Geometry check sheet. Reference: drawing and pictorial views, mm from the part's lowest x, y, z. Round coordinates to 2 decimals unless told otherwise and drop trailing zeros. Order: outer loops, then holes, each group sorted by start corner. A loop starts at its lowest first (then second) coordinate and runs counter-clockwise, first axis right, second up. Notation, with made-up numbers: (47, 43.5) -> (74, 43.5) arc R23 cw to (74, 58.5) -> close; hole circle Ø6 at (61.5, 40.5). An arc over 180 degrees is marked (long way). Put each result on its own line as item: value.
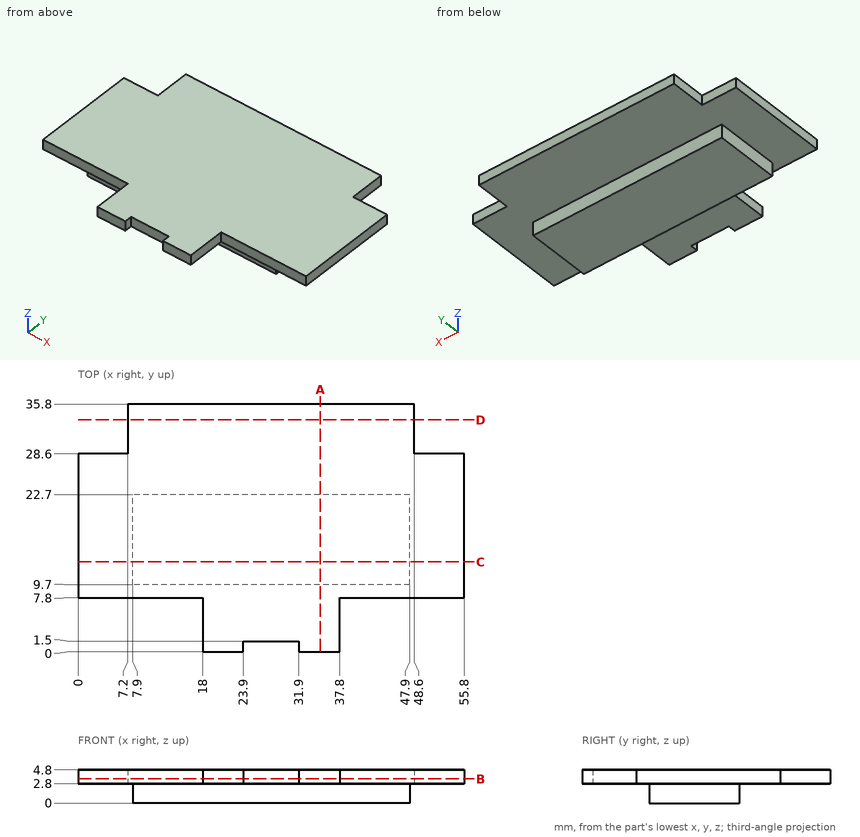
Item 1: Depth check by flat-ended pin: pin 1 Ø6 at (x, y) = (42, 15) entering from -Z; pin 2 Ø2 at (y, z) = (5.5, 3.5) entering from -X; pin 3 Ø1.6 at (y, z) = (3, 3.5) entering from +X; pin 4 Ø0.6 at (x, z) = (2, 4) entering from +Y. Enter the tip coordinate at first touch or a pass-through.
Geometry check:
pin 1: z = 0
pin 2: x = 18
pin 3: x = 37.8
pin 4: y = 28.6
Item 2: Sectioned sample at D-D, the plane y = 33.5. Record the boundary of the cut face in (x, z), then the cut area to 3 significant figures.
Geometry check:
outline: (7.2, 2.8) -> (48.6, 2.8) -> (48.6, 4.8) -> (7.2, 4.8) -> close
area: 82.8 mm2
Item 3: Material ranges on line 1 along Z through (x, y) = (29, 7); line 2 along Y through (x, z) = (38.5, 3.4); line 3 along X through (y, z) = (17.5, 1), recorded low to high.
Geometry check:
line 1: 2.8 to 4.8
line 2: 7.8 to 35.8
line 3: 7.9 to 47.9
Item 4: Sectioned sample at B-B, the plane z = 3.5. Record the boundary of the cut face in (x, y), then the cut area to 3 significant figures.
Geometry check:
outline: (0, 7.8) -> (18, 7.8) -> (18, 0) -> (23.9, 0) -> (23.9, 1.5) -> (31.9, 1.5) -> (31.9, 0) -> (37.8, 0) -> (37.8, 7.8) -> (55.8, 7.8) -> (55.8, 28.6) -> (48.6, 28.6) -> (48.6, 35.8) -> (7.2, 35.8) -> (7.2, 28.6) -> (0, 28.6) -> close
area: 1,600 mm2
Item 5: Sectioned sample at C-C, the plane y = 13. Record the boundary of the cut face in (x, z).
Geometry check:
outline: (0, 2.8) -> (7.9, 2.8) -> (7.9, 0) -> (47.9, 0) -> (47.9, 2.8) -> (55.8, 2.8) -> (55.8, 4.8) -> (0, 4.8) -> close
Item 6: Sectioned sample at A-A, the plane x = 35. Record the boundary of the cut face in (y, z), then the cut area to 3 significant figures.
Geometry check:
outline: (0, 2.8) -> (9.7, 2.8) -> (9.7, 0) -> (22.7, 0) -> (22.7, 2.8) -> (35.8, 2.8) -> (35.8, 4.8) -> (0, 4.8) -> close
area: 108 mm2
